from build123d import *

# Parameters (mm, degrees)
F0_W     = 30
F0_H     = 30
F1_DEPTH = 30
F3_DEPTH = 30.001
F5_R     = 5
F6_R     = 4.99999


# Not quite as in the source:
# - a fillet or chamfer is up to 0.001 mm smaller than in the source, because OpenCascade refuses the exact size


with BuildPart() as f1:
    # F0 (on Top) → F1 (new body)
    with BuildSketch(Plane.XY):
        with Locations((-170.8580559492, -194.9572271109)):
            Rectangle(F0_W, F0_H)
    extrude(amount=F1_DEPTH)

    # F2 (on face) → F3 (cut, through all)
    with BuildSketch(Plane.XZ.offset(209.9572271109)):
        with BuildLine():
            ThreePointArc((-170.8580559492, 20), (-174.3935898551, 11.4644660941), (-165.8580559492, 15))
            ThreePointArc((-165.8580559492, 15), (-167.3225220433, 18.5355339059), (-170.8580559492, 20))
        make_face()
    extrude(amount=-F3_DEPTH, mode=Mode.SUBTRACT)

    # F4: F1 across face


with BuildPart() as f1_1:
    add(f1.part)
    add(f1.part.mirror(Plane(origin=(-185.8580559492, -194.9572271109, 15), x_dir=(0, -1, 0), z_dir=(-1, 0, 0))))

    # F5
    f5_edges = [f1_1.edges().sort_by_distance(p)[0] for p in [
        (-215.858056, -209.957227, 15),
    ]]
    fillet(f5_edges, radius=F5_R)

    # F6 (radius 5 in the source; OpenCascade refuses exactly that, so slightly less here)
    f6_edges = [f1_1.edges().sort_by_distance(p)[0] for p in [
        (-215.858056, -179.957227, 15),
        (-195.858056, -209.957227, 15),
    ]]
    fillet(f6_edges, radius=F6_R)


solid = f1_1.part
Could you check a few things on this model? Use its own coordinates, in mm. Give positions to 0.01 mm unless a question says otherwise; leave off trailing zeros. Order: outer loops, then holes, each group sorted by start corner. A loop starts at its lowest first (then second) coordinate and runs counter-clockwise, first axis right, second up.
1. Suppose I cut it at B-B (z = 13). State how many separate pieces and enclosed holes the cut face has, plus the area to 3 significant figures.
Answers below:
separate pieces: 3
enclosed holes: 0
area: 1,230 mm2
2. I need wall thicknesses on L1, parallel to X at y = -201.25, z = 14.75; L2, parallel to Z at x = -200.5, y = -185.5; L3, parallel to X at y = -187.5, z = 15.75. Which ranges of each line are inside material? Lowest first, please.
Answers below:
L1: x = -215.86 to -205.85, -195.86 to -175.85, -165.86 to -155.86
L2: z = 0 to 10.01, 19.99 to 30
L3: x = -215.86 to -205.8, -195.91 to -175.8, -165.91 to -155.86
3. For pin 1 (11.5 mm diameter, centred on x = -170.86, z = 15, fed in from +Y); pin 2 (16 mm diameter, centred on x = -200.86, z = 15, fed in from -Y); pin 3 (6 mm diameter, centred on x = -172, z = 15.5, fed in from +Y), each with a flat end and sliding along its axis, tell me the tip position at first contact or that it passes through.
Answers below:
pin 1: stops at y = -179.96
pin 2: stops at y = -209.54
pin 3: passes through
4. Suppose I cut it at A-A (y = -189). Write out the boundary of the cut face in (x, z), plus the area to 3 significant figures.
Answers below:
outline: (-215.86, 0) - (-155.86, 0) - (-155.86, 30) - (-215.86, 30) - close; hole circle Ø10 at (-200.86, 15); hole circle Ø10 at (-170.86, 15)
area: 1,640 mm2
